Input: dimensioned drawing with shaded views. Units: mm. Origin: part minimum x, y, z. A direction names the side the tool comes from. Coordinates: 2 decimals unless noted, no trailing zeros. Order: outer loops, then holes, each group sorted by start corner. A loop starts at its lowest first (then second) coordinate and runs counter-clockwise, first axis right, second up. Notation, with made-up numbers: (83.25, 34) - (91.25, 34) arc R29 ccw to (91.25, 70) - close; hole circle Ø1 at (54, 30.25). An arc over 180 degrees is marked (long way). Answer as CSV lines item,"result". Start each with the question number.
Item 1: Draft query along Z for the marked faces 5, 6 and 7. Return one class per face: +Z half, -Z half, draft (parallel to the pull), parting line (faces both ways), or undercut.
Item 2: Material intervals for line 1 along Z through (x, y) = (1.4, 14.5); line 2 along Z through (x, y) = (5.45, 9.5); line 3 along Z through (x, y) = (3.85, 24), sorted ascending.
Item 3: Access query for the marked faces 1, 2, 3 and 4. Directions: +Z, -Z, +X, -X, +Y, -Y. A direction counts if a zero-diameter tool reaches every point of the face in a straight line with its end or side. Return the directions, or none.
Item 4: Section D-D (y = 24). Output: boundary loops of the cut face in (x, z).
Item 5: Section C-C (z = 24). Output: boundary loops of the cut face in (x, y).
Item 6: Section B-B (x = 5). Output: boundary loops of the cut face in (y, z).
Item 7: Section A-A (y = 14.5). Output: boundary loops of the cut face in (x, z), and give its area (3 significant figures).
Item 8: First-contact query: pin 1 (3 mm diameter, centred on x = 3.5, z = 35.5, fed in from -Y); pin 2 (0.5 mm diameter, centred on x = 4, z = 13, fed in from +Y); pin 3 (3 mm diameter, centred on x = 2, z = 34, fed in from +Y). Flat tips, straight axial feed; report the tip coordinate or a pass-through.
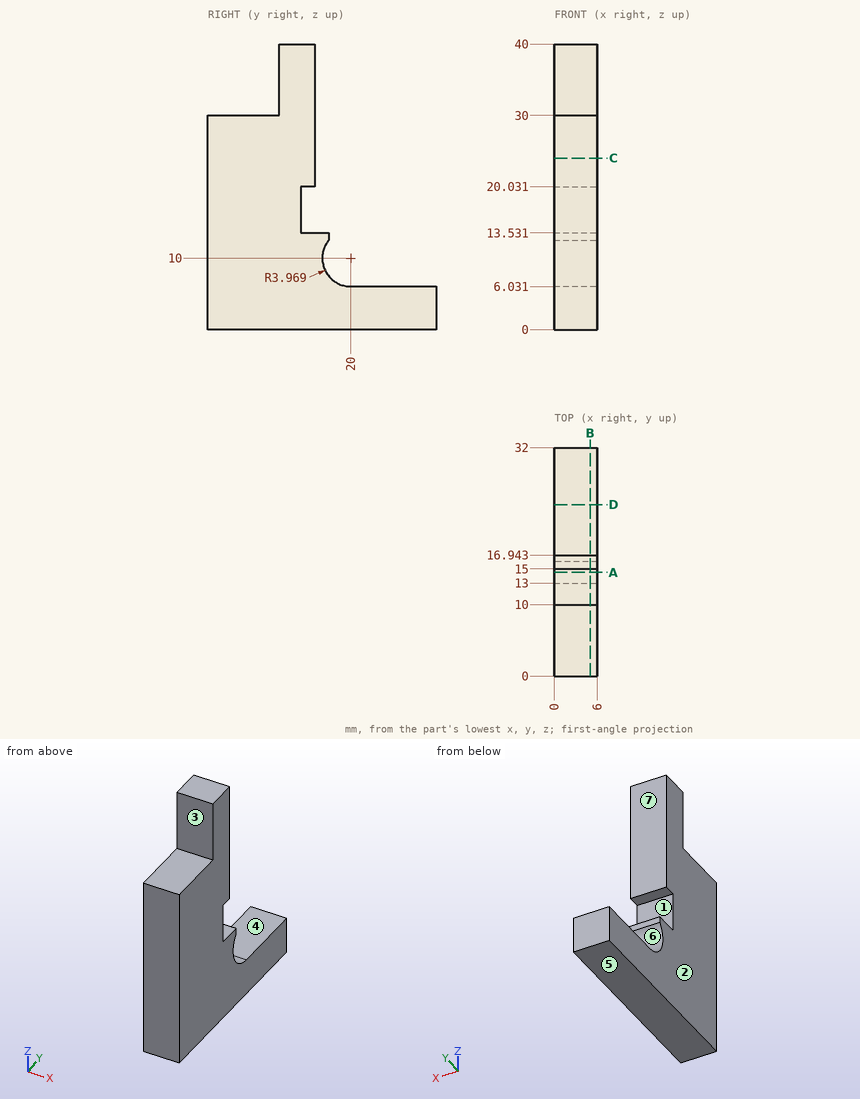
Determined:
1,face 5,"-Z half"
1,face 6,"undercut"
1,face 7,"draft"
2,line 1,"z = 0 to 13.53, 20.03 to 40"
2,line 2,"z = 0 to 30"
2,line 3,"z = 0 to 6.03"
3,face 1,"+X, -X, +Y"
3,face 2,"+Z, -Z, -X, +Y, -Y"
3,face 3,"+Z, +X, -X, -Y"
3,face 4,"+Z, +X, -X, +Y"
4,outline,"(0, 0) - (6, 0) - (6, 6.03) - (0, 6.03) - close"
5,outline,"(0, 0) - (6, 0) - (6, 15) - (0, 15) - close"
6,outline,"(0, 0) - (32, 0) - (32, 6.03) - (20, 6.03) arc R3.97 cw to (16.94, 12.53) - (16.94, 13.53) - (13, 13.53) - (13, 20.03) - (15, 20.03) - (15, 40) - (10, 40) - (10, 30) - (0, 30) - close"
7,outline,"(0, 0) - (6, 0) - (6, 13.53) - (0, 13.53) - close; (0, 20.03) - (6, 20.03) - (6, 40) - (0, 40) - close"
7,area,"201 mm^2"
8,pin 1,"stops at y = 10"
8,pin 2,"stops at y = 16.94"
8,pin 3,"stops at y = 15"
